```python
from build123d import *

# Parameters (mm, degrees)
F0_R     = 6.25
F0_R_2   = 2.6
F1_DEPTH = 7.5
F3_DEPTH = 5
F4_SIZE  = 0.5
F5_R     = 2.6
F6_DEPTH = 4


# Not quite as in the source:
# - a feature names something its author has since deleted; it is built from what else it names


with BuildPart() as f1:
    # F0 (on Top) → F1 (new body)
    with BuildSketch(Plane.XY):
        Circle(F0_R)
        Circle(F0_R_2, mode=Mode.SUBTRACT)
    extrude(amount=F1_DEPTH)

    # F2 (on face) → F3 (join, symmetric)
    with BuildSketch(Plane.XY.offset(7.5)):
        with BuildLine():
            Line((11, 2.5), (5.7282196187, 2.5))
            ThreePointArc((5.7282196187, 2.5), (6.1181644558, 1.2769352731), (6.25, 0))
            ThreePointArc((6.25, 0), (6.1181644558, -1.2769352731), (5.7282196187, -2.5))
            Line((5.7282196187, -2.5), (11, -2.5))
            ThreePointArc((11, -2.5), (12.0606601718, -2.0606601718), (12.5, -1))
            Line((12.5, -1), (12.5, 1))
            ThreePointArc((12.5, 1), (12.0606601718, 2.0606601718), (11, 2.5))
        make_face()
        with BuildLine():
            ThreePointArc((-5.7282196187, -2.5), (-6.25, 0), (-5.7282196187, 2.5))
            Line((-5.7282196187, 2.5), (-11, 2.5))
            ThreePointArc((-11, 2.5), (-12.0606601718, 2.0606601718), (-12.5, 1))
            Line((-12.5, 1), (-12.5, -1))
            ThreePointArc((-12.5, -1), (-12.0606601718, -2.0606601718), (-11, -2.5))
            Line((-11, -2.5), (-5.7282196187, -2.5))
        make_face()
        with BuildLine():
            ThreePointArc((6.25, 0), (6.1181644558, 1.2769352731), (5.7282196187, 2.5))
            ThreePointArc((5.7282196187, 2.5), (0, 6.25), (-5.7282196187, 2.5))
            ThreePointArc((-5.7282196187, 2.5), (-6.25, 0), (-5.7282196187, -2.5))
            ThreePointArc((-5.7282196187, -2.5), (0, -6.25), (5.7282196187, -2.5))
            ThreePointArc((5.7282196187, -2.5), (6.1181644558, -1.2769352731), (6.25, 0))
        make_face()
        Polygon((-4.1, 2.3671361037), (0, 4.7342722074), (4.1, 2.3671361037), (4.1, -2.3671361037), (0, -4.7342722074), (-4.1, -2.3671361037), align=None, mode=Mode.SUBTRACT)
    extrude(amount=F3_DEPTH, both=True)

    # F4
    f4_edges = [f1.edges().sort_by_distance(p)[0] for p in [
        (-6.25, 0, 0),
        (-2.6, 0, 0),
    ]]
    chamfer(f4_edges, length=F4_SIZE)

    # F5 (on face) → F6 (cut)
    with BuildSketch(Plane.XY.offset(7.5)):
        Polygon((4.1, -2.3671361037), (4.1, 2.3671361037), (0, 4.7342722074), (-4.1, 2.3671361037), (-4.1, -2.3671361037), (0, -4.7342722074), align=None)
        Circle(F5_R, mode=Mode.SUBTRACT)
    extrude(amount=-F6_DEPTH, mode=Mode.SUBTRACT)


solid = f1.part
```
The listing builds one solid part. Answer for the finished solid, in the listing's coordinates (mm). A direction names the side the tool comes from. Coordinates: 2 decimals unless noted, no trailing zeros. Loops run counter-clockwise (first coordinate to the right, second up) from the corner with the lowest first, then second, coordinate; pieces in that order, holes last. Notation, with made-up numbers: M 0.25,21 L 17.25,21 A27 cw 17.25,55 Z; hole C 66,22.5 d10. An arc over 180 degrees is marked long. Answer as a JSON object with one key per item and string values. Group by question number.
Item 1: Consider L1, parallel to Y at x = 0, z = 2; L2, parallel to Z at x = 6.75, y = 2; L3, parallel to X at y = 1, z = 9.25. Determine where each line is inside the solid, lowest interval first.
Item 2: Determine the mould class of faces 1 (the face through (-0.338, 2.578, 1.979)), 2 (the face through (-2, -2, 3.5)), 3 (the face through (9, 0, 2.5)), 4 (the face through (12.5, 0, 8)) for opening direction X: +X half, -X half, draft (parallel to the pull), parting line (faces both ways), or undercut.
Item 3: Section A-A (y = 0) is taken. Write down the section's boundary in (x, z).
Item 4: Each of these flat-tipped pins is pushed along its axis until it touches: P1, Ø2.5, axis at x = -10.5, y = 0.5, coming from the -Z side; P2, Ø4, axis at x = 0, y = 0, coming from the +Z side; P3, Ø1, axis at y = 3.5, z = 3, coming from the -X side; P4, Ø6, axis at x = 8.5, z = 8.5, coming from the +Y side. Where does it stop, or does it pass through?
Item 5: Section B-B (z = 8.5) is taken. Write down the section's boundary in (x, y), and give its area (3 significant figures).
Item 6: Which of the six approach directions +Z, -Z, +X, -X, +Y, -Y give full straight-line access (tool end or side, diameter ignored) to faces 5 (the face through (-8, 2.5, 8)), 6 (the face through (8, 2.5, 8)), 7 (the face through (-8, -2.5, 8)), 8 (the face through (8, -2.5, 8)), 9 (the face through (-2, 4, 12.5))?
Item 7: Section C-C (x = -6.75) is taken. Write down the section's boundary in (y, z).
Item 8: Section D-D (z = 1.75) is taken. Write down the section's boundary in (x, y).
Solved:
{
 "1": {"L1": "y = -6.25 to -2.6, 2.6 to 6.25", "L2": "z = 2.5 to 12.5", "L3": "x = -12.5 to -4.1, 4.1 to 12.5"},
 "2": {"face 1": "undercut", "face 2": "undercut", "face 3": "draft", "face 4": "+X half"},
 "3": {"outline": "M -12.5,2.5 L -6.25,2.5 L -6.25,0.5 L -5.75,0 L -3.1,0 L -2.6,0.5 L -2.6,3.5 L -4.1,3.5 L -4.1,12.5 L -12.5,12.5 Z; M 2.6,0.5 L 3.1,0 L 5.75,0 L 6.25,0.5 L 6.25,2.5 L 12.5,2.5 L 12.5,12.5 L 4.1,12.5 L 4.1,3.5 L 2.6,3.5 Z"},
 "4": {"P1": "stops at z = 2.5", "P2": "passes through", "P3": "stops at x = -5.48", "P4": "stops at y = 2.97"},
 "5": {"outline": "M -12.5,-1 A1.5 ccw -11,-2.5 L -5.73,-2.5 A6.25 ccw 5.73,-2.5 L 11,-2.5 A1.5 ccw 12.5,-1 L 12.5,1 A1.5 ccw 11,2.5 L 5.73,2.5 A6.25 ccw -5.73,2.5 L -11,2.5 A1.5 ccw -12.5,1 Z; hole M -4.1,-2.37 L 0,-4.73 L 4.1,-2.37 L 4.1,2.37 L 0,4.73 L -4.1,2.37 Z", "area": "127 mm2"},
 "6": {"face 5": "+Z, -Z, -X, +Y", "face 6": "+Z, -Z, +X, +Y", "face 7": "+Z, -Z, -X, -Y", "face 8": "+Z, -Z, +X, -Y", "face 9": "+Z, +X, -X, +Y, -Y"},
 "7": {"outline": "M -2.5,2.5 L 2.5,2.5 L 2.5,12.5 L -2.5,12.5 Z"},
 "8": {"outline": "C 0,0 d12.5; hole C 0,0 d5.2"}
}
